```python
from build123d import *

# Parameters (mm, degrees)
BOSS_EXTRUDE1_DEPTH      = 30.988
BOSS_EXTRUDE1_DEPTH_BACK = 30.988
SKETCH1_R                = 4
CUT_EXTRUDE1_START       = -4.000000101
CUT_EXTRUDE1_OUTLINE_R   = 1.500000048
CUT_EXTRUDE1_DEPTH       = 8.000000202
CHAMFER1_SIZE            = 0.56


# Read off the part's stored shape, not the designer's step: Cut-Extrude1
with BuildPart() as part:
    # Sketch1 → Boss-Extrude1 (new, two sides: drawn at the far end of the back side and taken through both)
    with BuildSketch(Plane.XY.offset(-BOSS_EXTRUDE1_DEPTH_BACK)):
        Circle(SKETCH1_R)
    extrude(amount=BOSS_EXTRUDE1_DEPTH + BOSS_EXTRUDE1_DEPTH_BACK)

    # Cut-Extrude1 outline → Cut-Extrude1 (cut)
    with BuildSketch(Plane.YZ.offset(CUT_EXTRUDE1_START)):
        with Locations((0, -19.812)):
            Circle(CUT_EXTRUDE1_OUTLINE_R)
    extrude(amount=CUT_EXTRUDE1_DEPTH, mode=Mode.SUBTRACT)

    # Chamfer1
    chamfer1_edges = [part.edges().sort_by_distance(p)[0] for p in [
        (-4, 0, -30.988),
        (-4, 0, 30.988),
    ]]
    chamfer(chamfer1_edges, length=CHAMFER1_SIZE)


solid = part.part
```
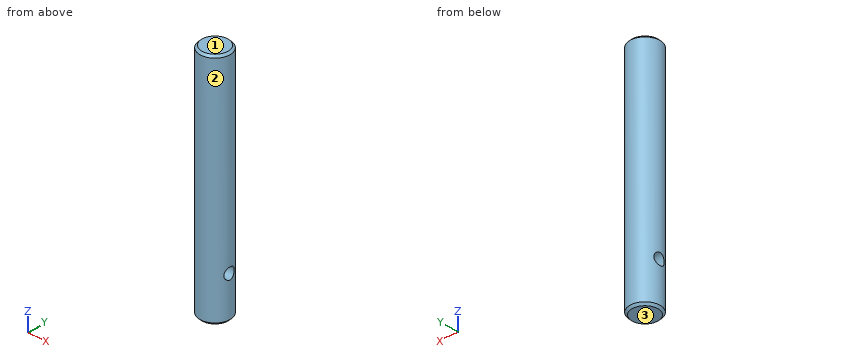
The listing builds one solid part. Answer for the finished solid, in the listing's coordinates (mm). Face numbers are marked on the shaded views. Give positions to 0.01 mm unless a question says otherwise; leave off trailing zeros. Loops run counter-clockwise (first coordinate to the right, second up) from the corner with the lowest first, then second, coordinate; pieces in that order, holes last. Notation, with made-up numbers: M 68,-38 L 102,-38 A18 cw 102,-16 Z; hole C 27,54 d5. An arc over 180 degrees is marked long. One line per item, written item: value.
Q1. Find the intervals of material crossed by line 1 (Z direction, x = 0, y = 0); line 2 (Z direction, x = 2, y = 0.75); line 3 (Y direction, x = 3.25, z = -19), in increasing order. Write a range as from..to.
Working result:
line 1: z = -30.99..-21.31, -18.31..30.99
line 2: z = -30.99..-21.11, -18.51..30.99
line 3: y = -2.33..-1.26, 1.26..2.33
Q2. A cutting plane is placed at A-A on y = 0. Determine the outline of the cut face in (x, z), then the cut area to 3 significant figures.
Working result:
outline: M -4,-30.43 L -3.44,-30.99 L 3.44,-30.99 L 4,-30.43 L 4,-21.31 L -4,-21.31 Z; M -4,-18.31 L 4,-18.31 L 4,30.43 L 3.44,30.99 L -3.44,30.99 L -4,30.43 Z
area: 471 mm^2
Q3. Flat-ended cylindrical pins translate along their axes: P1, Ø1.5, axis at x = 2.5, z = -21, coming from the +Y side; P2, Ø2, axis at y = 1.5, z = 23.5, coming from the -X side; P3, Ø3, axis at y = 3, z = -11, coming from the +X side. Find the tip coordinate at first contact, or state that the pin passes through.
Working result:
P1: stops at y = 3.6
P2: stops at x = -3.97
P3: stops at x = 3.71
Q4. A cutting plane is placed at B-B on x = 0. Determine the outline of the cut face in (y, z).
Working result:
outline: M -4,-30.43 L -3.44,-30.99 L 3.44,-30.99 L 4,-30.43 L 4,30.43 L 3.44,30.99 L -3.44,30.99 L -4,30.43 Z; hole C 0,-19.81 d3
Q5. Determine the mould class of the marked faces 1, 2 and 3 for opening direction Z: +Z half, -Z half, draft (parallel to the pull), parting line (faces both ways), or undercut.
Working result:
face 1: +Z half
face 2: draft
face 3: -Z half
Q6. A cutting plane is placed at C-C on z = 23.5. Determine the outline of the cut face in (x, y).
Working result:
outline: C 0,0 d8
